from build123d import *

# Parameters (mm, degrees)
SKIZZE1_W                       = 40
SKIZZE1_H                       = 235
AUFSATZ_LINEAR_AUSTRAGEN1_DEPTH = 10
SKIZZE2_R                       = 8
SCHNITT_LINEAR_AUSTRAGEN1_DEPTH = 120.608737139
VERRUNDUNG1_R                   = 10


with BuildPart() as part:
    # Skizze1 → Aufsatz-Linear austragen1 (new body)
    with BuildSketch(Plane(origin=(0, 0, 0), x_dir=(0, 0, -1), z_dir=(1, 0, 0))):
        Rectangle(SKIZZE1_W, SKIZZE1_H)
    extrude(amount=AUFSATZ_LINEAR_AUSTRAGEN1_DEPTH)

    # Skizze2 → Schnitt-Linear austragen1 (cut, through all)
    with BuildSketch(Plane(origin=(10, 0, 0), x_dir=(0, 0, -1), z_dir=(1, 0, 0))):
        with Locations((0, 105)):
            Circle(SKIZZE2_R)
        with Locations((0, -105)):
            Circle(SKIZZE2_R)
    extrude(amount=-SCHNITT_LINEAR_AUSTRAGEN1_DEPTH, mode=Mode.SUBTRACT)

    # Verrundung1
    verrundung1_edges = [part.edges().sort_by_distance(p)[0] for p in [
        (5, -117.5, -20),
        (5, 117.5, -20),
    ]]
    fillet(verrundung1_edges, radius=VERRUNDUNG1_R)


solid = part.part
Geometry check sheet. Reference: the model listing, model coordinates, mm. Coordinates: 2 decimals unless noted, no trailing zeros. Order: outer loops, then holes, each group sorted by start corner. A loop starts at its lowest first (then second) coordinate and runs counter-clockwise, first axis right, second up. Notation, with made-up numbers: (69, 38.25) -> (97, 38.25) arc R8 cw to (97, 46.25) -> close; hole circle Ø5 at (59, 24). An arc over 180 degrees is marked (long way). Use a Markdown table: item, result. Add a question column.
1. Cross-section at B-B (y = 105). Enter the section's corners in (x, z).
2. Material ranges on L1, parallel to Y at x = 7.75, z = 0; L2, parallel to Y at x = 2, z = 7; L3, parallel to Y at x = 1, z = -16, recorded low to high.
3. Cross-section at A-A (z = 0). Enter the section's corners in (x, y).
4. Cross-section at C-C (x = 1.5). Enter the section's corners in (y, z).
5. Mould release check, pull along Y, two halves, no side actions. Record for faces 1 (the face through (5.07, -114.65, -16.99)), 2 (the face through (5, -2, 20)), 3 (the face through (5.07, -112.81, 1.73)), 4 (the face through (5, 117.5, 5)): pulls with the +Y half, pulls with the -Y half, needs draft (parallel to the pull), parting line crosses it, or undercut.
Filled sheet:
| question | item | result |
|---|---|---|
| 1 | outline | (0, -20) -> (10, -20) -> (10, -8) -> (0, -8) -> close; (0, 8) -> (10, 8) -> (10, 20) -> (0, 20) -> close |
| 2 | L1 | -117.5 to -113, -97 to 97, 113 to 117.5 |
| 2 | L2 | -117.5 to -108.87, -101.13 to 101.13, 108.87 to 117.5 |
| 2 | L3 | -115.5 to 115.5 |
| 3 | outline | (0, -117.5) -> (10, -117.5) -> (10, -113) -> (0, -113) -> close; (0, -97) -> (10, -97) -> (10, 97) -> (0, 97) -> close; (0, 113) -> (10, 113) -> (10, 117.5) -> (0, 117.5) -> close |
| 4 | outline | (-117.5, -10) arc R10 ccw to (-107.5, -20) -> (107.5, -20) arc R10 ccw to (117.5, -10) -> (117.5, 20) -> (-117.5, 20) -> close; hole circle Ø16 at (-105, 0); hole circle Ø16 at (105, 0) |
| 5 | face 1 | pulls with the -Y half |
| 5 | face 2 | needs draft |
| 5 | face 3 | undercut |
| 5 | face 4 | pulls with the +Y half |
